```python
from build123d import *

# Parameters (mm, degrees)
F2_R          = 3.048
F3_DEPTH      = 76.2
F3_DEPTH_BACK = 76.2
F4_SIZE       = 1.27


with BuildPart() as f1:
    # F0 (on Front) → F1 (revolve)
    with BuildSketch(Plane.XZ):
        Polygon((50.8, 5.08), (0, 7.9375), (0, 6.731), (-20.609517, 6.731), (-20.609517, 0), (0, 0), (50.8, 0), align=None)
    revolve(axis=Axis((25.4, 0, 0), (-1, 0, 0)))

    # F2 (on Right) → F3 (cut, two sides)
    with BuildSketch(Plane.YZ) as f3_sk:
        Circle(F2_R)
    extrude(amount=F3_DEPTH, mode=Mode.SUBTRACT)
    extrude(f3_sk.sketch, amount=-F3_DEPTH_BACK, mode=Mode.SUBTRACT)

    # F4
    f4_edges = [f1.edges().sort_by_distance(p)[0] for p in [
        (50.8, 0, -5.08),
    ]]
    chamfer(f4_edges, length=F4_SIZE)


solid = f1.part
```
Can you work these out from the model? Positions are in its coordinate system, mm. A direction names the side the tool comes from. Give positions to 0.01 mm unless a question says otherwise; leave off trailing zeros. Loops run counter-clockwise (first coordinate to the right, second up) from the corner with the lowest first, then second, coordinate; pieces in that order, holes last. Notation, with made-up numbers: M 44.25,84 L 60.25,84 A30 ccw 60.25,110 Z; hole C -26.5,2.25 d2. An arc over 180 degrees is marked long. Use one line per item in the form item = value. Start each with the question number.
(1) On a 3-axis mill with a long thin cutter (end or side, diameter ignored), from which of +Z, -Z, +X, -X, +Y, -Y can I reach the whole of each face in a straight line? I mean faces 1 (the flat face through (-20.61, -1.4, 2.9)), 2 (the cylindrical face through (-10.45, -4.1, -5.34)). Say none if no direction works.
(2) I'm going to push flat-ended pins straight in: P1, Ø5, axis at y = 0, z = 0, coming from the +X side; P2, Ø1, axis at x = 31, y = -5.5, coming from the +Z side; P3, Ø5, axis at x = 29.5, z = -2.5, coming from the -Y side; P4, Ø5, axis at x = 29.5, z = -5, coming from the +Y side. Where does each tip first touch, or does it pass through?
(3) Please list where these lines run through material, in increasing order: line 1 (Z direction, x = 14, y = 0); line 2 (Y direction, x = 36.5, z = -2.75); line 3 (Z direction, x = -0.5, y = 6).
(4) I want a section at C-C, the plane x = 43.5. Write out the boundary of the cut face in (y, z).
(5) I want a section at A-A, the plane y = 0. Write out the boundary of the cut face in (x, z).
Worked out:
q1.face_1 = +Z, -Z, -X, +Y, -Y
q1.face_2 = -X
q2.P1 = through
q2.P2 = 3.66
q2.P3 = -6.34
q2.P4 = 5.77
q3.line_1 = -7.15 to -3.05, 3.05 to 7.15
q3.line_2 = -5.2 to -1.31, 1.31 to 5.2
q3.line_3 = -3.05 to 3.05
q4.outline = C 0,0 d10.98; hole C 0,0 d6.1
q5.outline = M -20.61,-6.73 L 0,-6.73 L 0,-7.94 L 49.53,-5.15 L 50.8,-3.81 L 50.8,-3.05 L -20.61,-3.05 Z; M -20.61,3.05 L 50.8,3.05 L 50.8,3.81 L 49.53,5.15 L 0,7.94 L 0,6.73 L -20.61,6.73 Z
